from build123d import *

# Parameters (mm, degrees)
BOSS_EXTRUDE1_DEPTH         = 3.175
F_1_4_0_25_DIAMETER_HOLE1_D = 6.35
F_1_4_CLEARANCE_HOLE1_D     = 6.7564


with BuildPart() as part:
    # Sketch1 → Boss-Extrude1 (new body)
    with BuildSketch(Plane(origin=(0, 0, 0), x_dir=(1, 0, 0), z_dir=(0, 1, 0))):
        Polygon((-462.534, 0), (-215.773, 449.26502653), (215.773, 449.26502653), (462.534, 0), align=None)
    extrude(amount=BOSS_EXTRUDE1_DEPTH)

    # 1/4 (0.25) Diameter Hole1 (through all)
    with Locations(Plane(origin=(0, 3.175, 0), x_dir=(1, 0, 0), z_dir=(0, 1, 0))):
        with Locations((-402.368285269, 83.160171278), (-255.632309055, 350.314795577), (-126.873, 436.56502653), (402.368285269, 83.160171278), (255.632309055, 350.314795577), (126.873, 436.56502653)):
            Hole(F_1_4_0_25_DIAMETER_HOLE1_D / 2)

    # 1/4 Clearance Hole1 (through all)
    with Locations(Plane(origin=(0, 3.175, 0), x_dir=(1, 0, 0), z_dir=(0, 1, 0))):
        with Locations((-376.682, 50.8), (-244.348, 50.8), (-123.952, 270.256), (-185.674, 398.526), (0, 224.79), (376.682, 50.8), (244.348, 50.8), (185.674, 398.526), (123.952, 270.256)):
            Hole(F_1_4_CLEARANCE_HOLE1_D / 2)


solid = part.part
The listing builds one solid part. Answer for the finished solid, in the listing's coordinates (mm). Coordinates: 2 decimals unless noted, no trailing zeros. Order: outer loops, then holes, each group sorted by start corner. A loop starts at its lowest first (then second) coordinate and runs counter-clockwise, first axis right, second up.
Q1. A cutting plane is placed at C-C, the plane x = -310. Write down the section's boundary in (y, z) (3 decimals), and give its area (3 significant figures).
Q2. A cutting plane is placed at A-A, the plane y = 2.45. State how many separate pieces and enclosed holes the cut face has, and give its area (3 significant figures).
Q3. A cutting plane is placed at B-B, the plane z = -257. Write down the section's boundary in (x, y) (1 decimal), and give its area (3 significant figures).
Q4. Consider line 1 (X direction, y = 2.95, z = -401); line 2 (Z direction, x = -127, y = 2.85); line 3 (X direction, y = 0.5, z = -397.5). Determine where each line is inside the solid, lowest interval first.
Answers follow:
1. outline: (0, -277.711) - (3.175, -277.711) - (3.175, 0) - (0, 0) - close
1. area: 882 mm2
2. separate pieces: 1
2. enclosed holes: 15
2. area: 304,000 mm2
3. outline: (-321.4, 0) - (321.4, 0) - (321.4, 3.2) - (-321.4, 3.2) - close
3. area: 2,040 mm2
4. line 1: x = -242.28 to -187.97, -183.37 to 183.37, 187.97 to 242.28
4. line 2: z = -449.27 to -439.74, -433.39 to -271.71, -268.8 to 0
4. line 3: x = -244.21 to -188.89, -182.46 to 182.46, 188.89 to 244.21
